Input: part model. Units: mm. Frame: model coordinates. A direction names the side the tool comes from. Coordinates: 2 decimals unless noted, no trailing zeros. Order: outer loops, then holes, each group sorted by start corner. A loop starts at its lowest first (then second) coordinate and runs counter-clockwise, first axis right, second up. Notation, with made-up numbers: M -3.5,6 L 50.5,6 A23 cw 50.5,37 Z; hole C 34,-21.5 d4. An arc over 180 degrees is marked long. One line per item, written item: value.
Autodesk Inventor part; units mm, degrees
ref_plane "Work Plane11" through (7.5, 24, 70) normal (0, 0, -1) x (-1, 0, 0)
ref_plane "YZ Plane" through (0, 0, 0) normal (1, 0, 0) x (0, 1, 0)
ref_plane "XZ Plane" through (0, 0, 0) normal (0, 1, 0) x (-1, 0, 0)
sketch "Sketch1" plane through (0, 0, 0) normal (0, 1, 0) x (-1, 0, 0)
  arc A0 (-8.9286, 8.7482) -> (8.9286, 8.7482) centre (0, 0) ccw
  line L0 (-7.5, 12.2474) -> (-7.5, 20)
  line L1 (7.5, 20) -> (7.5, 12.2474)
  line L2 (7.5, 20) -> (-7.5, 20)
  arc A1 (7.5, 12.2474) -> (8.9286, 8.7482) centre (12.5, 12.2474) ccw
  arc A2 (-8.9286, 8.7482) -> (-7.5, 12.2474) centre (-12.5, 12.2474) ccw
  point P0 (7.5, 10)
  point P1 (-7.5, 10)
  point P2 (0, 10)
  point P3 (0, 20)
  dimension "d0" = 25
  dimension "d109" = 5
  dimension "d129" = 15
  dimension "d131" = 10
extrude "Extrusion1" add sketch "Sketch1" against normal blind 12
sketch "Sketch22" plane through (-7.5, 0, 20) normal (0, 0, 1) x (1, 0, 0)
  line L0 (0, 0) -> (0, -12)
  line L1 (15, -12) -> (0, -12)
  line L2 (0, 0) -> (15, 0)
  line L3 (15, 0) -> (15, -12)
  line L4 (15, -12) -> (0, -12)
  line L5 (0, -12) -> (0, 0)
  point P0 (7.5, 0)
sketch "Sketch23" plane through (0, 0, 0) normal (1, 0, 0) x (0, 1, 0)
  line L0 (0, 20) -> (-12, 20)
  line L1 (-6, 20) -> (-6, 40)
  line L2 (24, 70) -> (134.0108, 70)
  arc A0 (24, 70) -> (-6, 40) centre (24, 40) ccw
  point P0 (0, 0)
  point P1 (-6, 70)
  dimension "d110" = 50
  dimension "d111" = 140.0108
  dimension "d112" = 90
  dimension "d113" = 30
sweep "Sweep2" add profiles "Sketch22" path "Sketch23" path curves L1 A0 L2
ref_plane "Work Plane11" through (7.5, 24, 70) normal (0, 0, -1) x (-1, 0, 0)
sketch "Sketch24" plane through (7.5, 24, 70) normal (0, 0, -1) x (-1, 0, 0)
  line L0 (0, 110.0108) -> (15, 110.0108)
  line L1 (0, 110.0108) -> (15, 110.0108)
  line L2 (0, 110.0108) -> (0, 113.964)
  line L3 (15, 110.0108) -> (15, 113.964)
  arc A0 (15, 113.964) -> (0, 113.964) centre (7.5, 122.0108) ccw
  line L4 (0, 110.0108) -> (15, 110.0108)
  point P0 (7.5, -24)
  point P1 (7.5, 110.0108)
  point P2 (7.5, 110.0108)
  dimension "d139" = 22
  dimension "d140" = 12
  dimension "d141" = 15
extrude "Extrusion17" add sketch "Sketch24" along normal mid plane 12
sketch "Sketch25" plane through (-7.5, 24, 76) normal (0, 0, 1) x (1, 0, 0)
  circle A0 centre (7.5, 122.0108) radius 2.5
  arc A1 (15, 113.964) -> (0, 113.964) centre (7.5, 122.0108) ccw
  point P0 (7.5, -24)
  dimension "d123" = 5
extrude "Extrusion18" cut sketch "Sketch25" against normal through all
sketch "Sketch27" plane through (0, 0, 0) normal (0, 1, 0) x (1, 0, 0)
  arc A0 (8.9286, -8.7482) -> (-8.9286, -8.7482) centre (0, 0) ccw
  circle A1 centre (0, 0) radius 2.4
  dimension "d136" = 4.8
extrude "Extrusion20" add sketch "Sketch27" against normal blind 26
sketch "Sketch28" plane through (7.5, 24, 64) normal (0, 0, -1) x (-1, 0, 0)
  circle A0 centre (7.5, 122.0108) radius 2.5
  circle A1 centre (7.5, 122.0108) radius 8.1
  point P0 (7.5, -24)
  dimension "d142" = 16.2
extrude "Extrusion21" cut sketch "Sketch28" against normal blind 5
mirror "Mirror2" about plane through (7.5, 24, 70) normal (0, 0, -1) of "Extrusion21"
sketch "Sketch29" plane through (0, 0, 0) normal (0, 1, 0) x (1, 0, 0)
  circle A0 centre (0, 0) radius 2.4
  line L0 (3.1754, 0) -> (1.5877, -2.75)
  line L1 (1.5877, -2.75) -> (-1.5877, -2.75)
  line L2 (-1.5877, -2.75) -> (-3.1754, 0)
  line L3 (-3.1754, 0) -> (-1.5877, 2.75)
  line L4 (-1.5877, 2.75) -> (1.5877, 2.75)
  line L5 (1.5877, 2.75) -> (3.1754, 0)
  dimension "d145" = 5.5
extrude "Extrusion22" cut sketch "Sketch29" against normal blind 3 contours A0 | L0 L1 L2 L3 L4 L5
sketch "Sketch30" plane through (0, -3, 0) normal (0, 1, 0) x (1, 0, 0)
  circle A0 centre (0, 0) radius 1.6
  dimension "d148" = 3.2
extrude "Extrusion23" cut sketch "Sketch30" against normal through all
properties part number "distal_link_2"
(1) Ray query, line 1 (X direction, y = -18.25, z = 0); line 2 (Y direction, x = 8, z = 6). Return the intervals inside material, ascending. Write a range as from..to.
Data:
line 1: x = -2.4..-1.6, 1.6..2.4
line 2: y = -12..0
(2) Cut plane B-B on z = 52. Output: boundary loops of the cut face in (x, y).
Data:
outline: M -7.5,-9.94 L 7.5,-9.94 L 7.5,3.22 L -7.5,3.22 Z
(3) Draft query along X for faces 4 (the cylindrical face through (-1.27, -14.34, 0.97)), 5 (the flat face through (7.5, 47, 65)), 6 (the flat face through (0, 91, 76)). Return one class per face: released by +X, released by -X, zero draft, split by the parting line, or undercut.
Data:
face 4: undercut
face 5: released by +X
face 6: zero draft
(4) Cut plane A-A on y = -5.5. Output: boundary loops of the cut face in (x, z).
Data:
outline: M -8.93,8.75 A12.5 ccw long 8.93,8.75 A5 cw 7.5,12.25 L 7.5,60.63 L -7.5,60.63 L -7.5,12.25 A5 cw Z; hole C 0,0 d3.2
(5) Cut plane C-C on y = 19. Output: boundary loops of the cut face in (x, z), plus the area to 3 significant figures.
Data:
outline: M -7.5,63.47 L 7.5,63.47 L 7.5,75.65 L -7.5,75.65 Z
area: 183 mm2
(6) Access query for faces 1 (the flat face through (0, 0, 13)), 2 (the cylindrical face through (1.054, 154.042, 66.465)), 3 (the flat face through (1.4, -3, -1.3)). Directions: +Z, -Z, +X, -X, +Y, -Y. A direction counts if a zero-diameter tool reaches every point of the face in a straight line with its end or side. Return the directions, or none.
Data:
face 1: -Z, +X, -X, +Y
face 2: -Z
face 3: +Y
(7) First-contact query: pin 1 (5 mm diameter, centred on x = 4, y = 148, fed in from -Z); pin 2 (6 mm diameter, centred on x = 5.5, z = 57, fed in from -Y); pin 3 (7.5 mm diameter, centred on x = -2, z = 4, fed in from +Y); pin 4 (4.5 mm diameter, centred on x = 0, y = 146.01, fed in from +Z). Flat tips, straight axial feed; report the tip coordinate or a pass-through.
Data:
pin 1: stops at z = 69
pin 2: stops at y = -9.17
pin 3: stops at y = 0
pin 4: passes through
